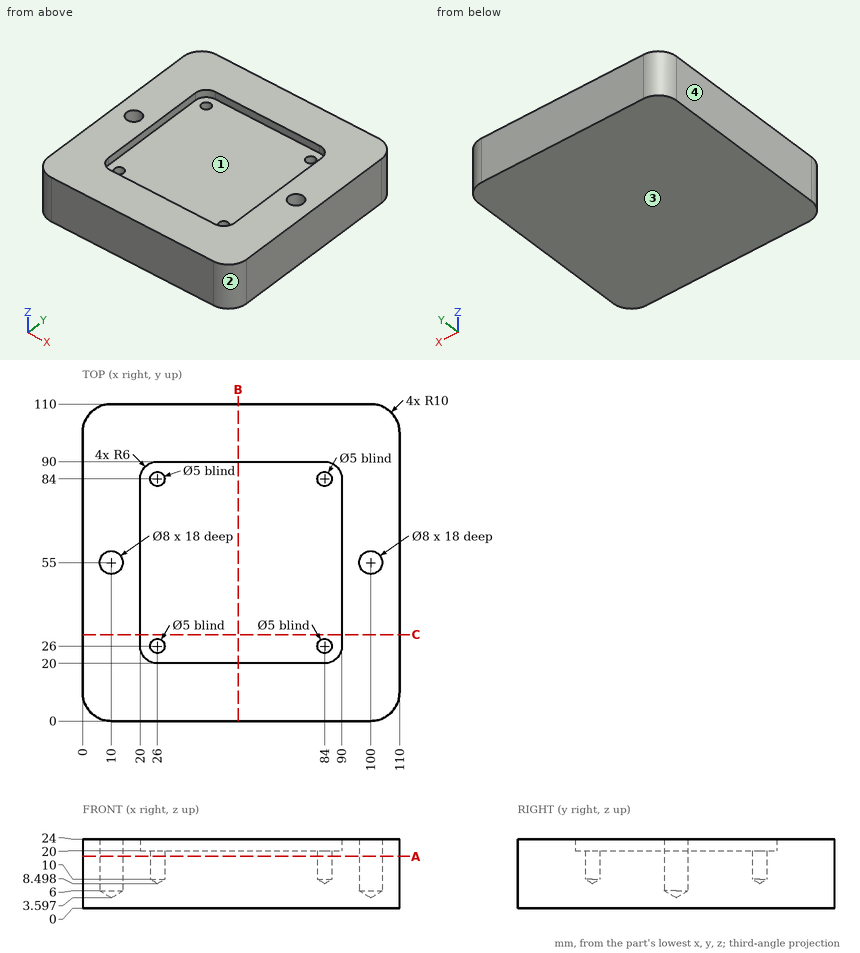
Drawing for the job (mm, zero at the part's lowest x, y, z). Give positions to 0.01 mm unless a question says otherwise; leave off trailing zeros. Loops run counter-clockwise (first coordinate to the right, second up) from the corner with the lowest first, then second, coordinate; pieces in that order, holes last.
(1) Band-saw the part on B-B (x = 54). Write the cut outline in (y, z), and give its area (3 significant figures).
Return value:
outline: (0, 0) - (110, 0) - (110, 24) - (90, 24) - (90, 20) - (20, 20) - (20, 24) - (0, 24) - close
area: 2,360 mm2
(2) Drill centre lines: line 1 along X through (y, z) = (26, 14); line 2 along X through (y, z) = (55, 19). Where is each one in solid material? Low to high.
Return value:
line 1: x = 0 to 23.5, 28.5 to 81.5, 86.5 to 110
line 2: x = 0 to 6, 14 to 96, 104 to 110
(3) Pull direction X, two halves, no side cores. Call the marked faces 1, 2, 3 and 4: pulls with the +X half, pulls with the -X half, needs draft (parallel to the pull), parting line crosses it, or undercut.
Return value:
face 1: undercut
face 2: pulls with the +X half
face 3: needs draft
face 4: pulls with the -X half
(4) Band-saw the part on A-A (z = 18). Write the cut outline in (x, y).
Return value:
outline: (0, 10) arc R10 ccw to (10, 0) - (100, 0) arc R10 ccw to (110, 10) - (110, 100) arc R10 ccw to (100, 110) - (10, 110) arc R10 ccw to (0, 100) - close; hole circle Ø8 at (10, 55); hole circle Ø5 at (26, 26); hole circle Ø5 at (26, 84); hole circle Ø5 at (84, 26); hole circle Ø5 at (84, 84); hole circle Ø8 at (100, 55)
(5) Pin check, flat tips, straight feed: pin 1 (21 mm diameter, centred on x = 42, y = 52, fed in from +Z); pin 2 (4.5 mm diameter, centred on x = 84, y = 26, fed in from +Z). Stop position of each tip, or through.
Return value:
pin 1: stops at z = 20
pin 2: stops at z = 9.85
